The model under review builds one solid part; all positions refer to its coordinate system, in mm. A direction names the side the tool comes from. Give positions to 0.01 mm unless a question says otherwise; leave off trailing zeros. Order: outer loops, then holes, each group sorted by start corner. A loop starts at its lowest first (then second) coordinate and runs counter-clockwise, first axis right, second up. Notation, with made-up numbers: (7.25, -26) - (47.25, -26) arc R23 cw to (47.25, -2) - close; hole circle Ø10 at (46, -1.5). An arc over 180 degrees is marked (long way). Use CSV: the item, a comma, the result in double quotes. Start each with the question number.
1. Machinability: for faces 1 (the flat face through (0, -11.748, 5)), 2 (the flat face through (33.21, -16, -4)), 3 (the flat face through (-33.02, 0, 8)), which of the approach directions +Z, -Z, +X, -X, +Y, -Y give a long, thin tool a straight path to every point of the face, cutting with its end or side? Answer none if there is none.
2. Draft analysis for pull direction X (two halves, no side actions). For faces 4 (the flat face through (40.068, 0, 1)), 5 (the cylindrical face through (-36.377, 16.254, 0.789)), 6 (the flat face through (-40.068, 0, 1)), state which applies: released by +X, released by -X, zero draft, split by the parting line, or undercut.
3. For pin 1 (1.3 mm diameter, centred on y = -15.5, z = -4.5, fed in from +X); pin 2 (2.5 mm diameter, centred on x = -37.78, y = 15.81, fed in from +Z); pin 3 (5.5 mm diameter, centred on x = 14.5, y = -0.5, fed in from +Z); pin 4 (5.5 mm diameter, centred on x = 7, z = 6.5, fed in from +Y), all flat-tipped, find the tip position at first contact; note any pin that passes through.
4. To check wall thickness, follow line 1 (Z direction, x = -23, y = -3); line 2 (Z direction, x = 34, y = 1); line 3 (Y direction, x = 35.5, z = 5.25). State the ranges of each line that lie inside material, in increasing order. Write a range as [from, to].
5. Take a section at B-B, the plane x = -20. State the section outline as (y, z) points.
6. Take a section at A-A, the plane y = -8. State the section outline as (x, z) points.
7. Take a section at D-D, the plane x = 1. State the section outline as (y, z) points.
8. Take a section at C-C, the plane z = 3. State the section outline as (x, y) points.
```python
from build123d import *

# Parameters (mm, degrees)
F0_W     = 80.137
F0_H     = 36.195
F0_R     = 1.4732
F1_DEPTH = 1.6002
F2_W     = 71.12
F2_H     = 23.9522
F3_DEPTH = 6.858
F4_T     = -2.54
F5_DEPTH = 4.572
F6_W     = 40.8432
F6_H     = 2.54
F7_DEPTH = 8.5598


with BuildPart() as f1:
    # F0 (on Top) → F1 (new body)
    with BuildSketch(Plane.XY):
        Rectangle(F0_W, F0_H)
        with Locations((-37.7825, -15.8115)):
            Circle(F0_R, mode=Mode.SUBTRACT)
        with Locations((37.7825, -15.8115)):
            Circle(F0_R, mode=Mode.SUBTRACT)
        with Locations((-37.7825, 15.8115)):
            Circle(F0_R, mode=Mode.SUBTRACT)
        with Locations((37.7825, 15.8115)):
            Circle(F0_R, mode=Mode.SUBTRACT)
    extrude(amount=F1_DEPTH)

    # F2 (on face) → F3 (join)
    with BuildSketch(Plane.XY.offset(1.6002)):
        with Locations((0, 0.2286)):
            Rectangle(F2_W, F2_H)
    extrude(amount=F3_DEPTH)

    # F4
    f4_openings = [f1.faces().sort_by_distance(p)[0] for p in [
        (0, 0.2286, 8.4582),
    ]]
    offset(amount=F4_T, openings=f4_openings)

    # F5 (add): a face of the model
    f5_faces = [f1.faces().sort_by_distance(p)[0] for p in [
        (0, 0.2286, 2.54),
    ]]
    extrude(f5_faces, amount=F5_DEPTH)

    # F6 (on face) → F7 (join)
    with BuildSketch(Plane(origin=(0, 0, 0), x_dir=(1, 0, 0), z_dir=(0, 0, -1))):
        with Locations((12.7889, 15.5575)):
            Rectangle(F6_W, F6_H)
    extrude(amount=F7_DEPTH)


solid = f1.part
```
Determined:
1,face 1,"+Z, +X, -X, -Y"
1,face 2,"-Z, +X, +Y, -Y"
1,face 3,"+Z"
2,face 4,"released by +X"
2,face 5,"undercut"
2,face 6,"released by -X"
3,pin 1,"stops at x = 33.21"
3,pin 2,"passes through"
3,pin 3,"stops at z = 7.11"
3,pin 4,"stops at y = 12.2"
4,line 1,"z = [0, 7.11]"
4,line 2,"z = [0, 8.46]"
4,line 3,"y = [-11.75, 12.2]"
5,outline,"(-18.1, 0) - (18.1, 0) - (18.1, 1.6) - (12.2, 1.6) - (12.2, 8.46) - (9.66, 8.46) - (9.66, 7.11) - (-9.21, 7.11) - (-9.21, 8.46) - (-11.75, 8.46) - (-11.75, 1.6) - (-18.1, 1.6) - close"
6,outline,"(-40.07, 0) - (40.07, 0) - (40.07, 1.6) - (35.56, 1.6) - (35.56, 8.46) - (33.02, 8.46) - (33.02, 7.11) - (-33.02, 7.11) - (-33.02, 8.46) - (-35.56, 8.46) - (-35.56, 1.6) - (-40.07, 1.6) - close"
7,outline,"(-18.1, 0) - (-16.83, 0) - (-16.83, -8.56) - (-14.29, -8.56) - (-14.29, 0) - (18.1, 0) - (18.1, 1.6) - (12.2, 1.6) - (12.2, 8.46) - (9.66, 8.46) - (9.66, 7.11) - (-9.21, 7.11) - (-9.21, 8.46) - (-11.75, 8.46) - (-11.75, 1.6) - (-18.1, 1.6) - close"
8,outline,"(-35.56, -11.75) - (35.56, -11.75) - (35.56, 12.2) - (-35.56, 12.2) - close"
